Can you work these out from the model? Positions are in its coordinate system, mm. A direction names the side the tool comes from. Round coordinates to 2 decimals unless told otherwise and drop trailing zeros. Loops run counter-clockwise (first coordinate to the right, second up) from the corner with the lowest first, then second, coordinate; pieces in that order, holes last. Notation, with made-up numbers: (22.25, 80) - (52.25, 80) arc R12 cw to (52.25, 96) - close; hole circle Ø2 at (68, 72.5). An arc over 180 degrees is marked (long way). Answer as CSV lines item,"result".
```python
from build123d import *

# Parameters (mm, degrees)
BOSS_EXTRUDE1_DEPTH = 11.1125
SKETCH6_R           = 3.5687
CUT_EXTRUDE1_DEPTH  = 7.62
SKETCH7_R           = 3.5687
CUT_EXTRUDE2_DEPTH  = 7.62


with BuildPart() as part:
    # Sketch1 → Boss-Extrude1 (new body, symmetric)
    with BuildSketch(Plane(origin=(0, -22.225, 0), x_dir=(0, -1, 0), z_dir=(-1, 0, 0))):
        with BuildLine():
            Line((0, 0), (0, 25.4))
            ThreePointArc((0, 25.4), (-3.367596045, 24.005096045), (-4.7625, 20.6375))
            Line((-4.7625, 20.6375), (-4.7625, 7.9375))
            ThreePointArc((-4.7625, 7.9375), (-5.69243597, 5.69243597), (-7.9375, 4.7625))
            Line((-7.9375, 4.7625), (-20.6375, 4.7625))
            ThreePointArc((-20.6375, 4.7625), (-24.005096045, 3.367596045), (-25.4, 0))
            Line((-25.4, 0), (0, 0))
        make_face()
    extrude(amount=BOSS_EXTRUDE1_DEPTH, both=True)

    # Sketch6 → Cut-Extrude1 (cut)
    with BuildSketch(Plane(origin=(0, -22.225, 0), x_dir=(-1, 0, 0), z_dir=(0, -1, 0))):
        with Locations((0, -12.7)):
            Circle(SKETCH6_R)
    extrude(amount=-CUT_EXTRUDE1_DEPTH, mode=Mode.SUBTRACT)

    # Sketch7 → Cut-Extrude2 (cut)
    with BuildSketch(Plane(origin=(0, 0, 0), x_dir=(-1, 0, 0), z_dir=(0, 0, -1))):
        with Locations((0, -9.525)):
            Circle(SKETCH7_R)
    extrude(amount=-CUT_EXTRUDE2_DEPTH, mode=Mode.SUBTRACT)


solid = part.part
```
Q1. Imagine slicing it at C-C (y = -7.5). Write out the boundary of the cut face in (x, z), then the cut area to 3 significant figures.
Checks:
outline,"(-11.11, 0) - (-2.94, 0) - (-2.94, 4.76) - (-11.11, 4.76) - close; (2.94, 0) - (11.11, 0) - (11.11, 4.76) - (2.94, 4.76) - close"
area,"77.9 mm²"
Q2. If I drill on line 1 along X through (y, z) = (-19.8, 12.7); line 2 along Y through (x, z) = (-3, 15.5) (1 decimal); line 3 along Z through (x, y) = (5.75, -14), over which ranges is the centre line in solid material (lowest first)? Write a range as [from, to].
Checks:
line 1,"[-11.11, -3.57], [3.57, 11.11]"
line 2,"[-22.2, -17.5]"
line 3,"[0, 4.76]"
Q3. On a 3-axis mill with a long thin cutter (end or side, diameter ignored), from which of +Z, -Z, +X, -X, +Y, -Y can I reach the whole of each face in a straight line? I mean faces 4 (the flat face through (0, -5, 4.762)), 5 (the flat face through (-3, -7, 0)). Say none if no direction works.
Checks:
face 4,"+Z, +X, -X, +Y"
face 5,"-Z, +X, -X, +Y, -Y"
Q4. Imagine slicing it at A-A (x = 0). Count the separate pieces of the cut face and the enclosed holes in it, then the cut area to 3 significant figures.
Checks:
separate pieces,"3"
enclosed holes,"0"
area,"144 mm²"
Q5. We'd pull the mould along X, two halves only. Please class faces 1 (the cylindrical face through (-1.65, -12.69, 2.35)), 2 (the flat face through (11.112, -15, 4)), 3 (the cylindrical face through (-0.16, -16.56, 5.72)): pulls with the +X half, pulls with the -X half, needs draft (parallel to the pull), parting line crosses it, or undercut.
Checks:
face 1,"undercut"
face 2,"pulls with the +X half"
face 3,"needs draft"
Q6. I'm going to push flat-ended pins straight in: pin 1 Ø10 at (x, z) = (-1, 11.5) entering from +Y; pin 2 Ø4 at (x, y) = (2.5, -9.5) entering from +Z; pin 3 Ø2 at (x, y) = (2, -15) entering from +Z. Where does each tip first touch, or does it pass through?
Checks:
pin 1,"y = -17.12"
pin 2,"z = 4.76"
pin 3,"z = 5.26"
Q7. Imagine slicing it at B-B (z = 12.7). Write out the boundary of the cut face in (x, y) (1 decimal), then the cut area to 3 significant figures.
Checks:
outline,"(-11.1, -22.2) - (-3.6, -22.2) - (-3.6, -17.5) - (-11.1, -17.5) - close; (3.6, -22.2) - (11.1, -22.2) - (11.1, -17.5) - (3.6, -17.5) - close"
area,"71.9 mm²"
